```python
from build123d import *

# Parameters (mm, degrees)
SKETCH1_W                                     = 50.8
SKETCH1_H                                     = 38.1
BODY_DEPTH                                    = 4.7625
CSK_FOR_8_FLAT_HEAD_MACHINE_SCREW1_AT_2_COUNT = 2
CSK_FOR_8_FLAT_HEAD_MACHINE_SCREW1_AT_2_PITCH = 30
CSK_FOR_8_FLAT_HEAD_MACHINE_SCREW2_AT_2_COUNT = 2
CSK_FOR_8_FLAT_HEAD_MACHINE_SCREW2_AT_2_PITCH = 9.525
FILLET1_R                                     = 2.54


with BuildPart() as part:
    # Sketch1 → Body (new body)
    with BuildSketch(Plane.XY):
        Rectangle(SKETCH1_W, SKETCH1_H)
    extrude(amount=BODY_DEPTH)

    # Sketch2 → CSK for #8 Flat Head Machine Screw1 (revolve, cut)
    with BuildSketch(Plane(origin=(-15, 0, 4.7625), x_dir=(0, -1, 0), z_dir=(1, 0, 0))):
        Polygon((0, 0), (0, 4.7625), (2.2479, 4.7625), (2.2479, 2.26450021), (4.2164, 0), align=None)
    csk_for_8_flat_head_machine_screw1 = revolve(axis=Axis((-15, 0, 11.1125), (0, 0, -1)), mode=Mode.SUBTRACT)

    # CSK for #8 Flat Head Machine Screw1 at 2: CSK for #8 Flat Head Machine Screw1 ×2
    with Locations(*[(i * CSK_FOR_8_FLAT_HEAD_MACHINE_SCREW1_AT_2_PITCH, 0, 0) for i in range(1, CSK_FOR_8_FLAT_HEAD_MACHINE_SCREW1_AT_2_COUNT)]):
        add(csk_for_8_flat_head_machine_screw1, mode=Mode.SUBTRACT)

    # Sketch3 → CSK for #8 Flat Head Machine Screw2 (revolve, cut)
    with BuildSketch(Plane.YZ.offset(4.7625)):
        Polygon((0, 0), (0, 4.7625), (2.2479, 4.7625), (2.2479, 2.26450021), (4.2164, 0), align=None)
    csk_for_8_flat_head_machine_screw2 = revolve(axis=Axis((4.7625, 0, -6.35), (0, 0, 1)), mode=Mode.SUBTRACT)

    # CSK for #8 Flat Head Machine Screw2 at 2: CSK for #8 Flat Head Machine Screw2 ×2
    with Locations(*[(-i * CSK_FOR_8_FLAT_HEAD_MACHINE_SCREW2_AT_2_PITCH, 0, 0) for i in range(1, CSK_FOR_8_FLAT_HEAD_MACHINE_SCREW2_AT_2_COUNT)]):
        add(csk_for_8_flat_head_machine_screw2, mode=Mode.SUBTRACT)

    # Fillet1
    fillet1_edges = [part.edges().sort_by_distance(p)[0] for p in [
        (-25.4, 0, 4.7625),
        (0, -19.05, 4.7625),
        (25.4, 0, 4.7625),
        (0, 19.05, 4.7625),
    ]]
    fillet(fillet1_edges, radius=FILLET1_R)


solid = part.part
```
Part model, mm, in its own coordinate system. Coordinates: 2 decimals unless noted, no trailing zeros. Loops run counter-clockwise (first coordinate to the right, second up) from the corner with the lowest first, then second, coordinate; pieces in that order, holes last. Notation, with made-up numbers: (59, 53) - (91, 53) arc R14 ccw to (91, 61) - close; hole circle Ø8 at (19.25, 54). An arc over 180 degrees is marked (long way). Write item = value, one per line. Start each with the question number.
Item 1: Cut at A-A, the plane y = 0. State how many separate pieces and enclosed holes the cut face has, and give its area (3 significant figures).
Item 2: Flat gauge pin, fed straight in: pin 1 Ø6 at (x, y) = (4.76, 0) entering from -Z. Where does the tip first touch, or does it go through?
Item 3: Cut at D-D, the plane x = 21.5. Give the cut face in (y, z), and give its area (3 significant figures).
Item 4: Mould opens along Y. For faces 1 (the cylindrical face through (0.356, -18.326, 3.999)), 2 (the flat face through (25.4, 0, 1)), 3 (the cylindrical face through (6.957, -0.487, 3.496)) say: released by +Y, released by -Y, zero draft, split by the parting line, or undercut.
Item 5: Cut at B-B, the plane x = 15. Give the cut face in (y, z), and give its area (3 significant figures).
Item 6: Wall check: L1, parallel to X at y = 1, z = 2.05; L2, parallel to X at y = 0, z = 2.9; L3, parallel to Y at x = -15, z = 0.75. Give the ranges that are in metal, low to high. Write a range as from..to.
Item 7: Cut at C-C, the plane z = 1.4. Give the cut face in (x, y), and give its area (3 significant figures).
The answers:
q1.separate_pieces = 5
q1.enclosed_holes = 0
q1.area = 136 mm2
q2.pin_1 = 1.4
q3.outline = (-19.05, 0) - (19.05, 0) - (19.05, 2.22) arc R2.54 ccw to (16.51, 4.76) - (-16.51, 4.76) arc R2.54 ccw to (-19.05, 2.22) - close
q3.area = 179 mm2
q4.face_1 = released by -Y
q4.face_2 = zero draft
q4.face_3 = undercut
q5.outline = (-19.05, 0) - (-2.25, 0) - (-2.25, 2.5) - (-4.22, 4.76) - (-16.51, 4.76) arc R2.54 ccw to (-19.05, 2.22) - close; (2.25, 0) - (19.05, 0) - (19.05, 2.22) arc R2.54 ccw to (16.51, 4.76) - (4.22, 4.76) - (2.25, 2.5) - close
q5.area = 153 mm2
q6.L1 = -25.4..-17.01, -12.99..-6.98, -2.54..2.54, 6.98..12.99, 17.01..25.4
q6.L2 = -25.31..-17.6, -12.4..-7.01, -2.51..2.51, 7.01..12.4, 17.6..25.31
q6.L3 = -19.05..-2.25, 2.25..19.05
q7.outline = (-25.4, -19.05) - (25.4, -19.05) - (25.4, 19.05) - (-25.4, 19.05) - close; hole circle Ø4.5 at (-15, 0); hole circle Ø6 at (-4.76, 0); hole circle Ø6 at (4.76, 0); hole circle Ø4.5 at (15, 0)
q7.area = 1,850 mm2
